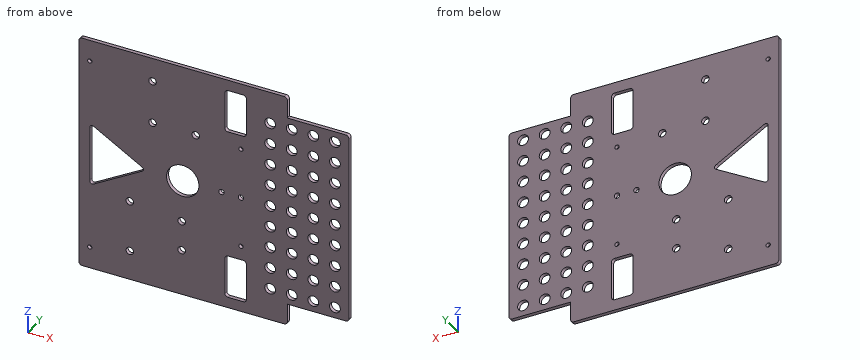
```python
from build123d import *

# Parameters (mm, degrees)
SKETCH1_W                       = 250
SKETCH1_H                       = 220
THE_UPPER_CHASISS_DEPTH         = 1.75
BATTARY_REACH                   = 168.517
SKETCH2_R                       = 2.5
BATTARY_DIRECTION_2_REACH       = 168.517
POWER_SECTION_REACH             = 168.517
SKETCH3_R                       = 3.5
POWER_SECTION_DIRECTION_2_REACH = 168.517
ARDUINO_R                       = 3.5
ARDUINO_SECTION_DEPTH           = 2.5
SKETCH7_R                       = 2
LINK_NAILS_DEPTH                = 5
SKETCH9_W                       = 20
SKETCH9_H                       = 40
RECT_CUT_DEPTH                  = 5
SKETCH10_R                      = 15
CIRC_CUT_DEPTH                  = 5
FILLET5_R                       = 3
SKETCH11_R                      = 5
CUT_EXTRUDE1_DEPTH              = 5
LPATTERN1_COUNT                 = 9
LPATTERN1_PITCH                 = 20
LPATTERN1_COUNT_DIR2            = 4
LPATTERN1_PITCH_DIR2            = 20
CUT_EXTRUDE2_DEPTH              = 5
CUT_EXTRUDE4_DEPTH              = 167.517454182
CUT_EXTRUDE4_DEPTH_BACK         = 167.517454182
FILLET7_R                       = 3


with BuildPart() as part:
    # Sketch1 → the upper chasiss (new, symmetric)
    with BuildSketch(Plane(origin=(0, 0, 0), x_dir=(1, 0, 0), z_dir=(0, 1, 0))):
        Rectangle(SKETCH1_W, SKETCH1_H)
    extrude(amount=THE_UPPER_CHASISS_DEPTH, both=True)

    # Battary: up to this face of the body (flat: up to its plane)
    battary_end = Plane(part.part.faces().sort_by_distance((0, 1.75, 0))[0])
    # Sketch2 → Battary (cut, up to the picked face)
    with BuildSketch(Plane(origin=(0, 0, 0), x_dir=(1, 0, 0), z_dir=(0, 1, 0)), mode=Mode.PRIVATE) as battary_sk1:
        with Locations(Location((25, 0, 0), (0, 0, 90))):
            Circle(SKETCH2_R)
    battary_tool1 = split(extrude(battary_sk1.sketch, amount=BATTARY_REACH, mode=Mode.PRIVATE), bisect_by=battary_end, keep=Keep.BOTH, mode=Mode.PRIVATE)
    # Sketch2 → Battary (cut, up to the picked face)
    with BuildSketch(Plane(origin=(0, 0, 0), x_dir=(1, 0, 0), z_dir=(0, 1, 0)), mode=Mode.PRIVATE) as battary_sk2:
        with Locations(Location((7, 0, 0), (0, 0, 90))):
            Circle(SKETCH2_R)
    battary_tool2 = split(extrude(battary_sk2.sketch, amount=BATTARY_REACH, mode=Mode.PRIVATE), bisect_by=battary_end, keep=Keep.BOTH, mode=Mode.PRIVATE)
    add(battary_tool1.solids().sort_by(Axis((25, 0, 0), (0, 1, 0)))[0], mode=Mode.SUBTRACT)
    add(battary_tool2.solids().sort_by(Axis((7, 0, 0), (0, 1, 0)))[0], mode=Mode.SUBTRACT)

    # Battary direction 2: up to this face of the body (flat: up to its plane)
    battary_direction_2_end = Plane(part.part.faces().sort_by_distance((0, -1.75, 0))[0])
    # Sketch2 → Battary direction 2 (cut, up to the picked face)
    with BuildSketch(Plane(origin=(0, 0, 0), x_dir=(1, 0, 0), z_dir=(0, 1, 0)), mode=Mode.PRIVATE) as battary_direction_2_sk1:
        with Locations(Location((25, 0, 0), (0, 0, 90))):
            Circle(SKETCH2_R)
    battary_direction_2_tool1 = split(extrude(battary_direction_2_sk1.sketch, amount=-BATTARY_DIRECTION_2_REACH, mode=Mode.PRIVATE), bisect_by=battary_direction_2_end, keep=Keep.BOTH, mode=Mode.PRIVATE)
    # Sketch2 → Battary direction 2 (cut, up to the picked face)
    with BuildSketch(Plane(origin=(0, 0, 0), x_dir=(1, 0, 0), z_dir=(0, 1, 0)), mode=Mode.PRIVATE) as battary_direction_2_sk2:
        with Locations(Location((7, 0, 0), (0, 0, 90))):
            Circle(SKETCH2_R)
    battary_direction_2_tool2 = split(extrude(battary_direction_2_sk2.sketch, amount=-BATTARY_DIRECTION_2_REACH, mode=Mode.PRIVATE), bisect_by=battary_direction_2_end, keep=Keep.BOTH, mode=Mode.PRIVATE)
    add(battary_direction_2_tool1.solids().sort_by(Axis((25, 0, 0), (0, -1, 0)))[0], mode=Mode.SUBTRACT)
    add(battary_direction_2_tool2.solids().sort_by(Axis((7, 0, 0), (0, -1, 0)))[0], mode=Mode.SUBTRACT)

    # power section: up to this face of the body (flat: up to its plane)
    power_section_end = Plane(part.part.faces().sort_by_distance((-0.011432136, -1.75, 0))[0])
    # Sketch3 → power section (cut, up to the picked face)
    with BuildSketch(Plane(origin=(0, 0, 0), x_dir=(1, 0, 0), z_dir=(0, 1, 0)), mode=Mode.PRIVATE) as power_section_sk1:
        with Locations(Location((-56.898371951, -47.760148577, 0), (0, 0, 90))):
            Circle(SKETCH3_R)
    power_section_tool1 = split(extrude(power_section_sk1.sketch, amount=-POWER_SECTION_REACH, mode=Mode.PRIVATE), bisect_by=power_section_end, keep=Keep.BOTH, mode=Mode.PRIVATE)
    # Sketch3 → power section (cut, up to the picked face)
    with BuildSketch(Plane(origin=(0, 0, 0), x_dir=(1, 0, 0), z_dir=(0, 1, 0)), mode=Mode.PRIVATE) as power_section_sk2:
        with Locations(Location((-16.898371951, -47.760148577, 0), (0, 0, 90))):
            Circle(SKETCH3_R)
    power_section_tool2 = split(extrude(power_section_sk2.sketch, amount=-POWER_SECTION_REACH, mode=Mode.PRIVATE), bisect_by=power_section_end, keep=Keep.BOTH, mode=Mode.PRIVATE)
    # Sketch3 → power section (cut, up to the picked face)
    with BuildSketch(Plane(origin=(0, 0, 0), x_dir=(1, 0, 0), z_dir=(0, 1, 0)), mode=Mode.PRIVATE) as power_section_sk3:
        with Locations(Location((-56.898371951, -87.760148577, 0), (0, 0, 90))):
            Circle(SKETCH3_R)
    power_section_tool3 = split(extrude(power_section_sk3.sketch, amount=-POWER_SECTION_REACH, mode=Mode.PRIVATE), bisect_by=power_section_end, keep=Keep.BOTH, mode=Mode.PRIVATE)
    add(power_section_tool1.solids().sort_by(Axis((-56.898372, 0, 47.760149), (0, -1, 0)))[0], mode=Mode.SUBTRACT)
    add(power_section_tool2.solids().sort_by(Axis((-16.898372, 0, 47.760149), (0, -1, 0)))[0], mode=Mode.SUBTRACT)
    add(power_section_tool3.solids().sort_by(Axis((-56.898372, 0, 87.760149), (0, -1, 0)))[0], mode=Mode.SUBTRACT)

    # power section direction 2: up to this face of the body (flat: up to its plane)
    power_section_direction_2_end = Plane(part.part.faces().sort_by_distance((-0.011432136, 1.75, 0))[0])
    # Sketch3 → power section direction 2 (cut, up to the picked face)
    with BuildSketch(Plane(origin=(0, 0, 0), x_dir=(1, 0, 0), z_dir=(0, 1, 0)), mode=Mode.PRIVATE) as power_section_direction_2_sk1:
        with Locations(Location((-56.898371951, -47.760148577, 0), (0, 0, 90))):
            Circle(SKETCH3_R)
    power_section_direction_2_tool1 = split(extrude(power_section_direction_2_sk1.sketch, amount=POWER_SECTION_DIRECTION_2_REACH, mode=Mode.PRIVATE), bisect_by=power_section_direction_2_end, keep=Keep.BOTH, mode=Mode.PRIVATE)
    # Sketch3 → power section direction 2 (cut, up to the picked face)
    with BuildSketch(Plane(origin=(0, 0, 0), x_dir=(1, 0, 0), z_dir=(0, 1, 0)), mode=Mode.PRIVATE) as power_section_direction_2_sk2:
        with Locations(Location((-16.898371951, -47.760148577, 0), (0, 0, 90))):
            Circle(SKETCH3_R)
    power_section_direction_2_tool2 = split(extrude(power_section_direction_2_sk2.sketch, amount=POWER_SECTION_DIRECTION_2_REACH, mode=Mode.PRIVATE), bisect_by=power_section_direction_2_end, keep=Keep.BOTH, mode=Mode.PRIVATE)
    # Sketch3 → power section direction 2 (cut, up to the picked face)
    with BuildSketch(Plane(origin=(0, 0, 0), x_dir=(1, 0, 0), z_dir=(0, 1, 0)), mode=Mode.PRIVATE) as power_section_direction_2_sk3:
        with Locations(Location((-56.898371951, -87.760148577, 0), (0, 0, 90))):
            Circle(SKETCH3_R)
    power_section_direction_2_tool3 = split(extrude(power_section_direction_2_sk3.sketch, amount=POWER_SECTION_DIRECTION_2_REACH, mode=Mode.PRIVATE), bisect_by=power_section_direction_2_end, keep=Keep.BOTH, mode=Mode.PRIVATE)
    add(power_section_direction_2_tool1.solids().sort_by(Axis((-56.898372, 0, 47.760149), (0, 1, 0)))[0], mode=Mode.SUBTRACT)
    add(power_section_direction_2_tool2.solids().sort_by(Axis((-16.898372, 0, 47.760149), (0, 1, 0)))[0], mode=Mode.SUBTRACT)
    add(power_section_direction_2_tool3.solids().sort_by(Axis((-56.898372, 0, 87.760149), (0, 1, 0)))[0], mode=Mode.SUBTRACT)

    # arduino → arduino section (cut, symmetric)
    with BuildSketch(Plane(origin=(0, 0, 0), x_dir=(1, 0, 0), z_dir=(0, 1, 0))):
        with Locations(Location((-77.933527642, 82.588848983, 0), (0, 0, 90))):
            Circle(ARDUINO_R)
        with Locations(Location((-77.933527642, 34.588848983, 0), (0, 0, 90))):
            Circle(ARDUINO_R)
        with Locations(Location((-29.933527642, 67.388848983, 0), (0, 0, 90))):
            Circle(ARDUINO_R)
        with Locations(Location((-29.933527642, 39.388848983, 0), (0, 0, 90))):
            Circle(ARDUINO_R)
    extrude(amount=ARDUINO_SECTION_DEPTH, both=True, mode=Mode.SUBTRACT)

    # Sketch7 → link nails (cut, symmetric)
    with BuildSketch(Plane(origin=(0, 1.75, 0), x_dir=(1, 0, 0), z_dir=(0, 1, 0))):
        with Locations(Location((-115, -90, 0), (0, 0, 90))):
            Circle(SKETCH7_R)
        with Locations(Location((-115, 90, 0), (0, 0, 90))):
            Circle(SKETCH7_R)
        with Locations(Location((25, 47, 0), (0, 0, 90))):
            Circle(SKETCH7_R)
        with Locations(Location((25, -47, 0), (0, 0, 90))):
            Circle(SKETCH7_R)
    extrude(amount=LINK_NAILS_DEPTH, both=True, mode=Mode.SUBTRACT)

    # Sketch9 → rect cut (cut, symmetric)
    with BuildSketch(Plane(origin=(0, 1.75, 0), x_dir=(1, 0, 0), z_dir=(0, 1, 0))):
        with Locations((20.066472358, 80)):
            Rectangle(SKETCH9_W, SKETCH9_H)
        with Locations((20.066472358, -80)):
            Rectangle(SKETCH9_W, SKETCH9_H)
    extrude(amount=RECT_CUT_DEPTH, both=True, mode=Mode.SUBTRACT)

    # Sketch10 → circ cut (cut, symmetric)
    with BuildSketch(Plane(origin=(0, 1.75, 0), x_dir=(1, 0, 0), z_dir=(0, 1, 0))):
        with Locations(Location((-28.923539072, 0, 0), (0, 0, 90))):
            Circle(SKETCH10_R)
    extrude(amount=CIRC_CUT_DEPTH, both=True, mode=Mode.SUBTRACT)

    # Fillet5
    fillet5_edges = [part.edges().sort_by_distance(p)[0] for p in [
        (10.066472358, 0, 100),
        (10.066472358, 0, 60),
        (30.066472358, 0, 60),
        (30.066472358, 0, 100),
        (30.066472358, 0, -100),
        (30.066472358, 0, -60),
        (10.066472358, 0, -60),
        (10.066472358, 0, -100),
    ]]
    fillet(fillet5_edges, radius=FILLET5_R)

    # Sketch11 → Cut-Extrude1 (cut, symmetric)
    with BuildSketch(Plane(origin=(0, 0, 0), x_dir=(1, 0, 0), z_dir=(0, 1, 0))):
        with Locations(Location((112, 80, 0), (0, 0, 90))):
            Circle(SKETCH11_R)
    cut_extrude1 = extrude(amount=CUT_EXTRUDE1_DEPTH, both=True, mode=Mode.SUBTRACT)

    # LPattern1: Cut-Extrude1 9 × 4
    with Locations(*[(-j * LPATTERN1_PITCH_DIR2, 0, i * LPATTERN1_PITCH) for i in range(LPATTERN1_COUNT) for j in range(LPATTERN1_COUNT_DIR2) if (i, j) != (0, 0)]):
        add(cut_extrude1, mode=Mode.SUBTRACT)

    # Sketch13 → Cut-Extrude2 (cut, symmetric)
    with BuildSketch(Plane(origin=(0, 0, 0), x_dir=(1, 0, 0), z_dir=(0, 1, 0))):
        Polygon((-115, 30), (-63.038475773, 0), (-115, -30), align=None)
    extrude(amount=CUT_EXTRUDE2_DEPTH, both=True, mode=Mode.SUBTRACT)

    # Fillet6
    # a fillet whose section is not a circle: 3 mm, written as the material it adds along each edge (its section moved 0.00015 mm through the faces so that the kernel can cut it)
    with BuildSketch(Plane(origin=(-115, -1.75, 30), x_dir=(0.8660398371803181, 0, -0.4999749997916777), z_dir=(0, 1, 0)), Plane(origin=(-63.038475773, 1.75, 0), x_dir=(-0.8660109696668712, 0, 0.500024999791656), z_dir=(0, -1, 0)), Plane(origin=(-115, -1.75, -30), x_dir=(-2.8867513448411456e-05, 0, 0.9999999995833333), z_dir=(0, 1, 0))) as fillet6_piece_1:
        with BuildLine():
            add(Edge.make_bspline([(5.196152425, 0), (4.416690591, -2.2501e-05), (3.637228756, -4.5002e-05), (1.991685226, 0.449929995), (1.385406821, 1.499964994), (1.818393539, 3.150059994), (2.20810497, 3.825104994), (2.5978164, 4.500149994)], knots=[0, 0, 0, 0, 0, 0, 0.5, 0.5, 1, 1, 1, 1, 1, 1], degree=5))
            Line((2.5978164, 4.500149994), (2.54585401, 4.530148494))
            ThreePointArc((2.54585401, 4.530148494), (1.247010763, 2.280035999), (-0.05196239, 0.0299985))
            Line((-0.05196239, 0.0299985), (1.732e-06, -0.06))
            ThreePointArc((1.732e-06, -0.06), (2.598077942, -0.059925), (5.196154157, -0.06))
            Line((5.196154157, -0.06), (5.196152425, 0))
        make_face()
    extrude(amount=3.5)

    # Sketch16 → Cut-Extrude4 (cut, two sides: drawn at the far end of the back side and taken through both)
    with BuildSketch(Plane(origin=(0, 0, 0), x_dir=(1, 0, 0), z_dir=(0, 1, 0)).offset(-CUT_EXTRUDE4_DEPTH_BACK)):
        Polygon((68, 705.317008407), (68, 110), (68, 90), (125, 90), (125, -90), (68, -90), (68, -110), (68, -705.317008407), (1258.634016814, -705.317008407), (1258.634016814, 705.317008407), align=None)
    extrude(amount=CUT_EXTRUDE4_DEPTH + CUT_EXTRUDE4_DEPTH_BACK, mode=Mode.SUBTRACT)

    # Fillet7
    fillet7_edges = [part.edges().sort_by_distance(p)[0] for p in [
        (125, 0, 90),
        (68, 0, 110),
        (125, 0, -90),
        (68, 0, -110),
        (-125, 0, 110),
        (-125, 0, -110),
    ]]
    fillet(fillet7_edges, radius=FILLET7_R)


solid = part.part
```
Check sheet for the modelled part. Datum: model origin and axes. Units: mm. Round coordinates to 2 decimals unless told otherwise and drop trailing zeros. Write each loop counter-clockwise with the first axis right and the second up, starting at its lowest first coordinate (ties: lowest second). Pieces come first, ordered by that corner, then holes. Notation, with made-up numbers: (43.5, 72.25) -> (53.5, 72.25) arc R12 ccw to (53.5, 86.25) -> close; hole circle Ø8 at (-24.75, 52.25). An arc over 180 degrees is marked (long way). One line per question, with ' | ' between items. Start each with the question number.
1. Sectioned sample at B-B, the plane z = 72. Record the cut outline in (x, y), then the cut area to 3 significant figures.
2. Depth check by flat-ended pin: pin 1 (1 mm diameter, centred on x = 96, y = -0.5, fed in from +Z). Enter the tip coordinate at first touch or a pass-through.
3. Scan lines: line 1 along X through (y, z) = (0.55, 40); line 2 along X through (y, z) = (0.5, 80); line 3 along X through (y, z) = (0.5, 97). Record each from-to range of solid material in increasing order. Write a range as from..to.
4. Sectioned sample at A-A, the plane z = 40. Record the cut outline in (x, y), then the cut area to 3 significant figures.
5. Sectioned sample at C-C, the plane x = -97. Record the cut outline in (y, z), then the cut area to 3 significant figures.
6. Sectioned sample at D-D, the plane z = -8. Record the cut outline in (x, y).
Taken from the geometry:
1) outline: (-125, -1.75) -> (10.07, -1.75) -> (10.07, 1.75) -> (-125, 1.75) -> close; (30.07, -1.75) -> (125, -1.75) -> (125, 1.75) -> (30.07, 1.75) -> close | area: 805 mm^2
2) pin 1: stops at z = 90
3) line 1: x = -125..47, 57..67, 77..87, 97..107, 117..125 | line 2: x = -125..10.07, 30.07..47, 57..67, 77..87, 97..107, 117..125 | line 3: x = -125..10.07, 30.07..68
4) outline: (-125, -1.75) -> (47, -1.75) -> (47, 1.75) -> (-125, 1.75) -> close; (57, -1.75) -> (67, -1.75) -> (67, 1.75) -> (57, 1.75) -> close; (77, -1.75) -> (87, -1.75) -> (87, 1.75) -> (77, 1.75) -> close; (97, -1.75) -> (107, -1.75) -> (107, 1.75) -> (97, 1.75) -> close; (117, -1.75) -> (125, -1.75) -> (125, 1.75) -> (117, 1.75) -> close | area: 735 mm^2
5) outline: (-1.75, -110) -> (1.75, -110) -> (1.75, -19.61) -> (-1.75, -19.61) -> close; (-1.75, 19.61) -> (1.75, 19.61) -> (1.75, 110) -> (-1.75, 110) -> close | area: 633 mm^2
6) outline: (-125, -1.75) -> (-115, -1.75) -> (-115, 1.75) -> (-125, 1.75) -> close; (-76.89, -1.75) -> (-41.61, -1.75) -> (-41.61, 1.75) -> (-76.89, 1.75) -> close; (-16.23, -1.75) -> (125, -1.75) -> (125, 1.75) -> (-16.23, 1.75) -> close
